from build123d import *

# Parameters (mm, degrees)
BOSS_EXTRUDE1_DEPTH = 98.425
SKETCH2_R           = 3.175
CUT_EXTRUDE1_DEPTH  = 12.7
FILLET1_R           = 6.35


with BuildPart() as part:
    # Sketch1 → Boss-Extrude1 (new body, symmetric)
    with BuildSketch(Plane.XY):
        with BuildLine():
            Line((44.45, 9.525), (50.8, 9.525))
            Line((50.8, 9.525), (50.8, 3.175))
            Line((50.8, 3.175), (50.8, -3.175))
            Line((50.8, -3.175), (50.8, -9.525))
            Line((50.8, -9.525), (44.45, -9.525))
            Line((44.45, -9.525), (-44.45, -9.525))
            ThreePointArc((-44.45, -9.525), (-48.940128061, -7.665128061), (-50.8, -3.175))
            Line((-50.8, -3.175), (-50.8, 3.175))
            ThreePointArc((-50.8, 3.175), (-48.940128061, 7.665128061), (-44.45, 9.525))
            Line((-44.45, 9.525), (44.45, 9.525))
        make_face()
    extrude(amount=BOSS_EXTRUDE1_DEPTH, both=True)

    # Sketch2 → Cut-Extrude1 (cut)
    with BuildSketch(Plane.XY.offset(98.425)):
        with Locations((-25.4, 0)):
            Circle(SKETCH2_R)
        with Locations((25.4, 0)):
            Circle(SKETCH2_R)
    cut_extrude1 = extrude(amount=-CUT_EXTRUDE1_DEPTH, mode=Mode.SUBTRACT)

    # Fillet1
    fillet1_edges = [part.edges().sort_by_distance(p)[0] for p in [
        (50.8, -9.525, 0),
        (50.8, 9.525, 0),
    ]]
    fillet(fillet1_edges, radius=FILLET1_R)

    # Mirror1: Cut-Extrude1 across plane
    add(cut_extrude1.mirror(Plane.XY), mode=Mode.SUBTRACT)


solid = part.part
Geometry check sheet. Reference: the model listing, model coordinates, mm. A direction names the side the tool comes from. Give positions to 0.01 mm unless a question says otherwise; leave off trailing zeros. Order: outer loops, then holes, each group sorted by start corner. A loop starts at its lowest first (then second) coordinate and runs counter-clockwise, first axis right, second up. Notation, with made-up numbers: (65, 59.25) - (104, 59.25) arc R17 cw to (104, 87.25) - close; hole circle Ø4 at (89, 20). An arc over 180 degrees is marked (long way). Answer as a JSON object with one key per item and string values.
(1) Draft check along X on faces 1 (the flat face through (-1, 9.525, 1)), 2 (the cylindrical face through (-48.89, -7.714, 1.378)), 3 (the flat face through (-25, 0, -85.725)), 4 (the cylindrical face through (48.989, 7.615, 1.378)). Enter one of: released by +X, released by -X, zero draft, split by the parting line, or undercut.
Report:
{"face 1": "zero draft", "face 2": "released by -X", "face 3": "undercut", "face 4": "released by +X"}
(2) Tool access check on faces 5 (the cylindrical face through (28.43, 0.95, 92.16)), 6 (the flat face through (25, 0, -85.725)), 7 (the flat face through (1, 0, -98.425)). Record the directions out of +Z, -Z, +X, -X, +Y, -Y that give a thin tool (end or side, any length) a straight path to the whole face; none if there is none.
Report:
{"face 5": "+Z", "face 6": "-Z", "face 7": "-Z, +X, -X, +Y, -Y"}
(3) Cross-section at B-B (z = -49). Record the cut outline in (x, y) (3 decimals).
Report:
{"outline": "(-50.8, -3.175) arc R6.35 ccw to (-44.45, -9.525) - (44.45, -9.525) arc R6.35 ccw to (50.8, -3.175) - (50.8, 3.175) arc R6.35 ccw to (44.45, 9.525) - (-44.45, 9.525) arc R6.35 ccw to (-50.8, 3.175) - close"}
(4) Depth check by flat-ended pin: pin 1 Ø4 at (x, y) = (-25.4, 0) entering from -Z (3 decimals); pin 2 Ø4 at (y, z) = (-5.5, 1) entering from -X; pin 3 Ø3 at (x, y) = (25.5, -0.5) entering from +Z (3 decimals). Enter the tip coordinate at first touch or a pass-through.
Report:
{"pin 1": "z = -85.725", "pin 2": "x = -50.79", "pin 3": "z = 85.725"}
(5) Cross-section at A-A (x = 25.4). Record the cut outline in (y, z) (3 decimals).
Report:
{"outline": "(-9.525, -98.425) - (-3.175, -98.425) - (-3.175, -85.725) - (3.175, -85.725) - (3.175, -98.425) - (9.525, -98.425) - (9.525, 98.425) - (3.175, 98.425) - (3.175, 85.725) - (-3.175, 85.725) - (-3.175, 98.425) - (-9.525, 98.425) - close"}
(6) Material ranges on line 1 (Y direction, x = -25, z = -90) (3 decimals); line 2 (Y direction, x = -25.4, z = -91) (3 decimals); line 3 (X direction, y = -2.25, z = -88), recorded low to high.
Report:
{"line 1": "-9.525 to -3.15, 3.15 to 9.525", "line 2": "-9.525 to -3.175, 3.175 to 9.525", "line 3": "-50.8 to -27.64, -23.16 to 23.16, 27.64 to 50.8"}
(7) Cross-section at C-C (x = -26.5). Record the cut outline in (y, z) (3 decimals).
Report:
{"outline": "(-9.525, -98.425) - (-2.978, -98.425) - (-2.978, -85.725) - (2.978, -85.725) - (2.978, -98.425) - (9.525, -98.425) - (9.525, 98.425) - (2.978, 98.425) - (2.978, 85.725) - (-2.978, 85.725) - (-2.978, 98.425) - (-9.525, 98.425) - close"}
